```python
from build123d import *

# Parameters (mm, degrees)
SKETCH1_R           = 50.8
SKETCH1_R_2         = 16.129
BOSS_EXTRUDE1_DEPTH = 1.5875
CIRPATTERN1_COUNT   = 6


with BuildPart() as part:
    # Sketch1 → Boss-Extrude1 (new body)
    with BuildSketch(Plane.XY):
        Circle(SKETCH1_R)
        Circle(SKETCH1_R_2, mode=Mode.SUBTRACT)
    extrude(amount=BOSS_EXTRUDE1_DEPTH)

    # Sketch2 → 3/32 (0.09375) Diameter Hole1 (revolve, cut)
    with BuildSketch(Plane(origin=(0, 19.05, 1.5875), x_dir=(0, -1, 0), z_dir=(1, 0, 0))):
        Polygon((0, 0), (0, 26.115399675), (1.190625, 25.4), (1.190625, 0), align=None)
    f_3_32_0_09375_diameter_hole1 = revolve(axis=Axis((0, 19.05, 7.9375), (0, 0, -1)), mode=Mode.SUBTRACT)

    # CirPattern1: 3/32 (0.09375) Diameter Hole1 ×6 about axis
    cirpattern1_axis = Axis((0, 0, 0), (0, 0, 1))
    for i in range(1, CIRPATTERN1_COUNT):
        add(f_3_32_0_09375_diameter_hole1.rotate(cirpattern1_axis, i * 360 / CIRPATTERN1_COUNT), mode=Mode.SUBTRACT)


solid = part.part
```
Can you work these out from the model? Positions are in its coordinate system, mm. Round coordinates to 2 decimals unless told otherwise and drop trailing zeros. Loops run counter-clockwise (first coordinate to the right, second up) from the corner with the lowest first, then second, coordinate; pieces in that order, holes last. Notation, with made-up numbers: M 50.5,13 L 63.5,13 A38 cw 63.5,51 Z; hole C 22.25,73 d5. An arc over 180 degrees is marked long. Answer as a JSON object with one key per item and string values. Group by question number.
Q1. Imagine slicing it at D-D, the plane z = 1.3. Please give me the cut outline in (x, y) (3 decimals).
Q2. Please list where these lines run through material, in increasing order: L1, parallel to Y at x = 0, z = 0.6; L2, parallel to Y at x = 6.5, z = 0.55; L3, parallel to X at y = 4.5, z = 0.75.
Q3. Imagine slicing it at A-A, the plane y = 0. Please give me the cut outline in (x, z), then the cut area to 3 significant figures.
Q4. Will this pin go through, and if not, where does the flat tip stop? pin 1 (3 mm diameter, centred on x = 0, y = -19.05, fed in from -Z).
Q5. We'd pull the mould along Y, two halves only. Please class faces 1 (the cylindrical face through (16.954, -10.625, 0.805)), 2 (the cylindrical face through (-11.012, -49.592, 0.783)), 3 (the flat face through (-12, 12, 1.588)): +Y half, -Y half, draft (parallel to the pull), parting line (faces both ways), or undercut.
Q6. Imagine slicing it at C-C, the plane x = -12. Please give me the cut outline in (y, z), then the cut area to 3 significant figures.
Q7. Imagine slicing it at B-B, the plane x = 0. Please give me the cut outline in (y, z), then the cut area to 3 significant figures.
Findings:
{
 "1": {"outline": "C 0,0 d101.6; hole C -16.498,-9.525 d2.381; hole C -16.498,9.525 d2.381; hole C 0,0 d32.258; hole C 0,-19.05 d2.381; hole C 0,19.05 d2.381; hole C 16.498,-9.525 d2.381; hole C 16.498,9.525 d2.381"},
 "2": {"L1": "y = -50.8 to -20.24, -17.86 to -16.13, 16.13 to 17.86, 20.24 to 50.8", "L2": "y = -50.38 to -14.76, 14.76 to 50.38", "L3": "x = -50.6 to -15.49, 15.49 to 50.6"},
 "3": {"outline": "M -50.8,0 L -16.13,0 L -16.13,1.59 L -50.8,1.59 Z; M 16.13,0 L 50.8,0 L 50.8,1.59 L 16.13,1.59 Z", "area": "110 mm2"},
 "4": {"pin 1": "stops at z = 0"},
 "5": {"face 1": "undercut", "face 2": "parting line", "face 3": "draft"},
 "6": {"outline": "M -49.36,0 L -10.78,0 L -10.78,1.59 L -49.36,1.59 Z; M 10.78,0 L 49.36,0 L 49.36,1.59 L 10.78,1.59 Z", "area": "123 mm2"},
 "7": {"outline": "M -50.8,0 L -20.24,0 L -20.24,1.59 L -50.8,1.59 Z; M -17.86,0 L -16.13,0 L -16.13,1.59 L -17.86,1.59 Z; M 16.13,0 L 17.86,0 L 17.86,1.59 L 16.13,1.59 Z; M 20.24,0 L 50.8,0 L 50.8,1.59 L 20.24,1.59 Z", "area": "103 mm2"}
}
